Design review of the part built by this model. Coordinates are the model's own, in mm. Face numbers are marked on the shaded views. Give positions to 0.01 mm unless a question says otherwise; leave off trailing zeros. Order: outer loops, then holes, each group sorted by start corner. A loop starts at its lowest first (then second) coordinate and runs counter-clockwise, first axis right, second up. Notation, with made-up numbers: (-0.5, 14.5) -> (7.5, 14.5) arc R18 ccw to (7.5, 23.5) -> close; hole circle Ø3 at (36, -18.75). An arc over 180 degrees is marked (long way). Return JSON: item names as keys, results as strings.
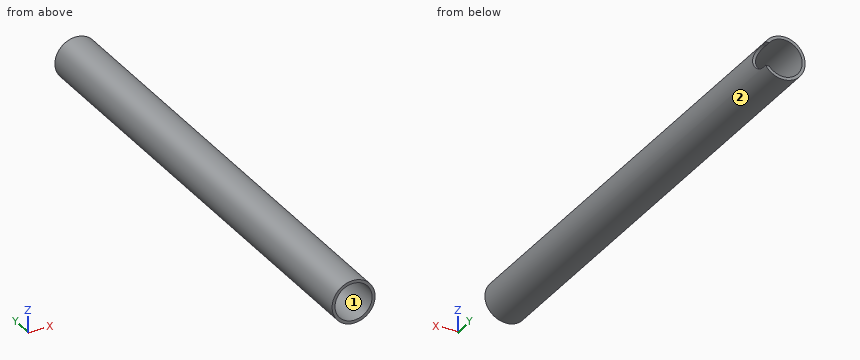
Autodesk Inventor part; units mm, degrees
ref_plane "Work Plane1" through (11, 0, 0) normal (1, 0, 0) x (0, 1, 0)
ref_plane "XZ Plane" through (0, 0, 0) normal (0, 1, 0) x (-1, 0, 0)
ref_plane "XY Plane" through (0, 0, 0) normal (0, 0, 1) x (1, 0, 0)
sketch "Sketch1" plane through (0, 0, 0) normal (0, 0, 1) x (1, 0, 0)
  line L0 (0, 0) -> (0, 260)
  line L1 (0, 260) -> (11, 260)
  line L2 (11, 260) -> (11, 0)
  line L3 (11, 0) -> (0, 0)
  dimension "d0" = 22
  dimension "d1" = 260
revolve "Revolution1" add sketch "Sketch1" angle 360 about axis through (0, 0, 0) along (0, 1, 0)
sketch "Sketch2" plane through (0, 0, 0) normal (0, -1, 0) x (1, 0, 0)
  circle A0 centre (0, 0) radius 11
hole "Hole1" at (0, 0, 0) direction (0, 1, 0) diameter 19 depth 260
ref_plane "Work Plane1" through (11, 0, 0) normal (1, 0, 0) x (0, 1, 0)
sketch "Sketch3" plane through (11, 0, 0) normal (1, 0, 0) x (0, 1, 0)
  line L0 (260, -11) -> (260, 11)
  line L1 (0, -11) -> (0, 11)
  line L2 (0, -11) -> (260, -11)
  line L3 (0, 11) -> (260, 11)
  line L4 (260, -6) -> (257, -6)
  arc A0 (257, 6) -> (257, -6) centre (257, 0) ccw
  line L5 (257, 6) -> (260, 6)
  point P0 (0, 0)
  point P1 (0, 0)
  dimension "d11" = 3
  dimension "d12" = 6
extrude "Extrusion1" cut sketch "Sketch3" against normal up to surface contours L4 A0 L5 L0
properties part number "132 part 1" material "Aluminum 6061-AHC"
Item 1: Wall thickness on L1, parallel to X at y = 193.5, z = 0; L2, parallel to Z at x = -2, y = 234: over which ranges is each line inside the solid? List them lowest first. Write a range as [from, to].
Result set:
{"L1": "x = [-11, -9.5], [9.5, 11]", "L2": "z = [-10.82, -9.29], [9.29, 10.82]"}
Item 2: For pin 1 (8 mm diameter, centred on x = -5.5, y = 81.5, fed in from -Z); pin 2 (4 mm diameter, centred on y = 215, z = 7.5, fed in from -X); pin 3 (6 mm diameter, centred on x = -6, y = 212.5, fed in from +Z); pin 4 (6 mm diameter, centred on x = 3, y = 148, fed in from -Z), all flat-tipped, find the tip position at first contact; note any pin that passes through.
Result set:
{"pin 1": "stops at z = -10.9", "pin 2": "stops at x = -9.53", "pin 3": "stops at z = 10.58", "pin 4": "stops at z = -11"}
Item 3: Add section A-A (x = 0). Give the boundary of the cut face in (y, z), plus the area to 3 significant figures.
Result set:
{"outline": "(0, -11) -> (260, -11) -> (260, -9.5) -> (0, -9.5) -> close; (0, 9.5) -> (260, 9.5) -> (260, 11) -> (0, 11) -> close", "area": "780 mm^2"}
Item 4: Add section C-C (y = 228). Give the boundary of the cut face in (x, z), plus the area to 3 significant figures.
Result set:
{"outline": "circle Ø22 at (0, 0); hole circle Ø19 at (0, 0)", "area": "96.6 mm^2"}
Item 5: Add section B-B (z = 0). Give the boundary of the cut face in (x, y).
Result set:
{"outline": "(-11, 0) -> (-9.5, 0) -> (-9.5, 260) -> (-11, 260) -> close; (9.5, 0) -> (11, 0) -> (11, 251) -> (9.5, 251) -> close"}
Item 6: Mouldability with a two-part tool opening along Z and no side actions: class the marked faces 1 and 2 as released by +Z, released by -Z, zero draft, split by the parting line, or undercut.
Result set:
{"face 1": "undercut", "face 2": "split by the parting line"}
